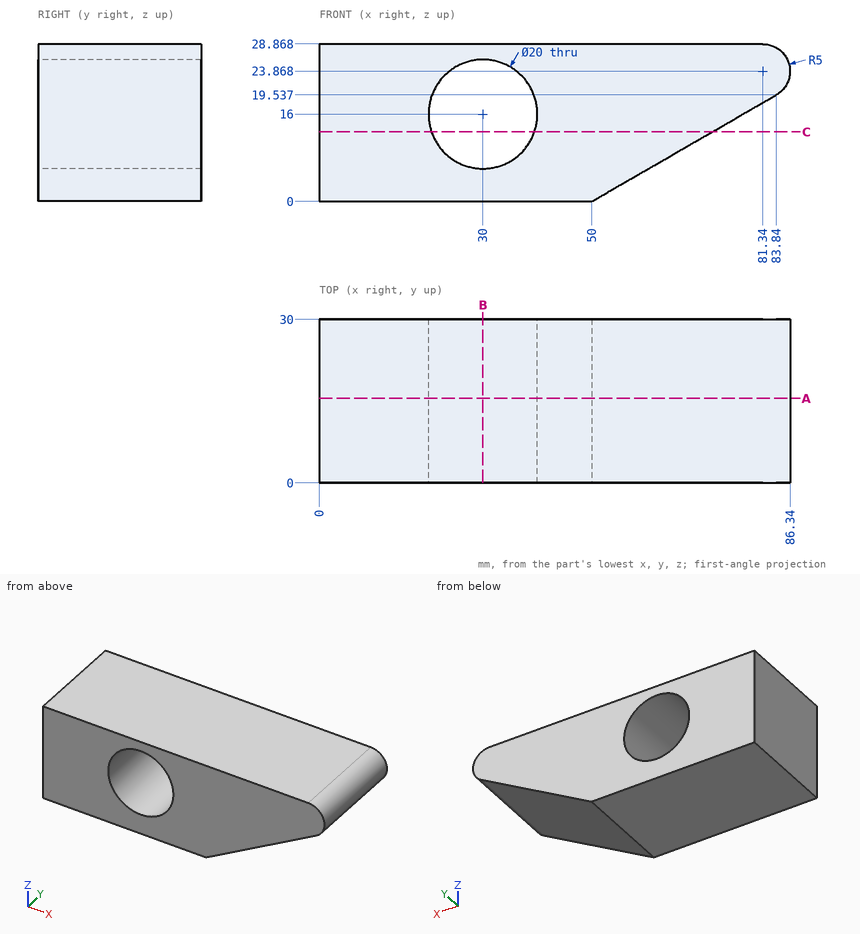
Can you work these out from the drawing? Everything is in mm from the part's minimum corner. Coordinates: 2 decimals unless noted, no trailing zeros. Loops run counter-clockwise (first coordinate to the right, second up) from the corner with the lowest first, then second, coordinate; pieces in that order, holes last.
1) Imagine slicing it at A-A on y = 15.5. List the corners of the cut face in (x, z) for me, plus the area to 3 significant figures.
2) For pin 1 (12 mm diameter, centred on y = 12.5, z = 6, fed in from -X); pin 2 (1.5 mm diameter, centred on y = 24.5, z = 17, fed in from +X) (1 decimal), each with a flat end and sliding along its axis, tell me the tip position at first contact or that it passes through.
3) I need wall thicknesses on probe 1 along Z at (x, y) = (30, 13.25); probe 2 along X at (y, z) = (4, 12.75) (1 decimal); probe 3 along X at (y, z) = (9, 25) (1 decimal). Which ranges of each line are inside material? Lowest first, please.
4) Imagine slicing it at B-B on x = 30. List the corners of the cut face in (y, z) for me.
5) Imagine slicing it at C-C on z = 12.75. List the corners of the cut face in (x, y) for me.
Completed:
1. outline: (0, 0) - (50, 0) - (83.84, 19.54) arc R5 ccw to (81.34, 28.87) - (0, 28.87) - close; hole circle Ø20 at (30, 16)
1. area: 1,790 mm2
2. pin 1: stops at x = 0
2. pin 2: stops at x = 80.7
3. probe 1: z = 0 to 6, 26 to 28.87
3. probe 2: x = 0 to 20.5, 39.5 to 72.1
3. probe 3: x = 0 to 25.6, 34.4 to 86.2
4. outline: (0, 0) - (30, 0) - (30, 6) - (0, 6) - close; (0, 26) - (30, 26) - (30, 28.87) - (0, 28.87) - close
5. outline: (0, 0) - (20.54, 0) - (20.54, 30) - (0, 30) - close; (39.46, 0) - (72.08, 0) - (72.08, 30) - (39.46, 30) - close
